CAD build for the part. Positions are in the model's coordinates, mm. Coordinates: 2 decimals unless noted, no trailing zeros. Loops run counter-clockwise (first coordinate to the right, second up) from the corner with the lowest first, then second, coordinate; pieces in that order, holes last. Notation, with made-up numbers: (-38, 23) - (-17, 23) arc R9 cw to (-17, 38) - close; hole circle Ø3 at (78.25, -8). An arc over 180 degrees is marked (long way). Put each result on its own line as item: value.
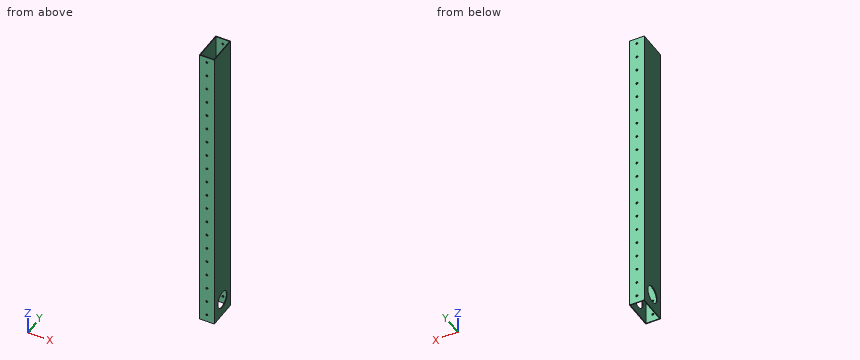
Autodesk Inventor part; units mm, degrees
ref_plane "YZ Plane" through (0, 0, 0) normal (1, 0, 0) x (0, 1, 0)
ref_plane "XZ Plane" through (0, 0, 0) normal (0, 1, 0) x (-1, 0, 0)
ref_plane "XY Plane" through (0, 0, 0) normal (0, 0, 1) x (1, 0, 0)
sketch "Sketch1" plane through (0, 0, 0) normal (0, 0, 1) x (1, 0, 0)
  line L0 (-12.1708, 16.0073) -> (13.2292, 16.0073)
  line L1 (13.2292, 16.0073) -> (13.2292, -34.7927)
  line L2 (13.2292, -34.7927) -> (-12.1708, -34.7927)
  line L3 (-12.1708, -34.7927) -> (-12.1708, 16.0073)
  line L4 (11.9592, 14.7373) -> (-10.9008, 14.7373)
  line L5 (-10.9008, 14.7373) -> (-10.9008, -33.5227)
  line L6 (-10.9008, -33.5227) -> (11.9592, -33.5227)
  line L7 (11.9592, -33.5227) -> (11.9592, 14.7373)
  point P0 (0, 0)
  dimension "d0" = 25.4
  dimension "d1" = 50.8
  dimension "d2" = 1.27
extrude "Extrusion1" add sketch "Sketch1" along normal blind 504.825
sketch "Sketch2" plane through (-12.1708, 16.0073, 0) normal (0, 1, 0) x (1, 0, 0)
  circle A0 centre (12.7, -12.7) radius 1.7272
  line L0 (25.4, 0) -> (0, 0)
  line L1 (0, 0) -> (0, -504.825)
  point P0 (12.1708, 0)
  dimension "d5" = 3.4544
  dimension "d6" = 12.7
  dimension "d7" = 12.7
extrude "Extrusion2" cut sketch "Sketch2" against normal through all
pattern_linear "Rectangular Pattern1" count 50 spacing 25.4 along (0, 0, 1) of "Extrusion2"
sketch "Sketch5" plane through (13.2292, -34.7927, 0) normal (1, 0, 0) x (0, 0, -1)
  line L0 (-504.825, 0) -> (-504.825, 50.8)
  line L1 (0, 50.8) -> (-504.825, 50.8)
  circle A0 centre (-28.575, 25.4) radius 14.2875
  line L2 (0, 0) -> (-504.825, 0)
  point P0 (0, 34.7927)
  dimension "d52" = 28.575
  dimension "d54" = 25.4
  dimension "d62" = 25.4
  dimension "d63" = 28.575
extrude "Extrusion5" cut sketch "Sketch5" against normal through all
equation "\"d3\" = d13"
equation "\"d10\" = d14"
equation "\"d13\" = 504.825"
equation "\"d14\" = d13"
equation "\"d32\" = 101.6"
properties part number "AIntakeSupport2"
Q1. Wall check: L1, parallel to X at y = -14.5, z = 377; L2, parallel to Y at x = 2.25, z = 180; L3, parallel to X at y = -34.45, z = 342.9. Give the ranges that are in metal, low to high. Write a range as from..to.
Determined:
L1: -12.17..-10.9, 11.96..13.23
L2: -34.79..-33.52, 14.74..16.01
L3: -12.17..-1.2, 2.26..13.23
Q2. Slice it at B-B, the plane z = 47. Give the cut face in (x, y).
Determined:
outline: (-12.17, -34.79) - (13.23, -34.79) - (13.23, 16.01) - (-12.17, 16.01) - close; hole (-10.9, -33.52) - (11.96, -33.52) - (11.96, 14.74) - (-10.9, 14.74) - close
Q3. Slice it at A-A, the plane x = -6. Give the cut face in (y, z) (3 decimals).
Determined:
outline: (-34.793, 0) - (-33.523, 0) - (-33.523, 504.825) - (-34.793, 504.825) - close; (14.737, 0) - (16.007, 0) - (16.007, 504.825) - (14.737, 504.825) - close
Q4. Slice it at C-C, the plane y = -19.5. Give the cut face in (x, z) (3 decimals).
Determined:
outline: (-12.171, 0) - (-10.901, 0) - (-10.901, 18.477) - (-12.171, 18.477) - close; (-12.171, 38.673) - (-10.901, 38.673) - (-10.901, 504.825) - (-12.171, 504.825) - close; (11.959, 0) - (13.229, 0) - (13.229, 18.477) - (11.959, 18.477) - close; (11.959, 38.673) - (13.229, 38.673) - (13.229, 504.825) - (11.959, 504.825) - close
